Input: part model. Units: mm. Frame: model coordinates. Face numbers are marked on the shaded views. A direction names the side the tool comes from. Coordinates: 2 decimals unless noted, no trailing zeros. Write each loop counter-clockwise with the first axis right and the second up, starting at its lowest first coordinate (ties: lowest second). Pieces come first, ordered by that corner, then holes.
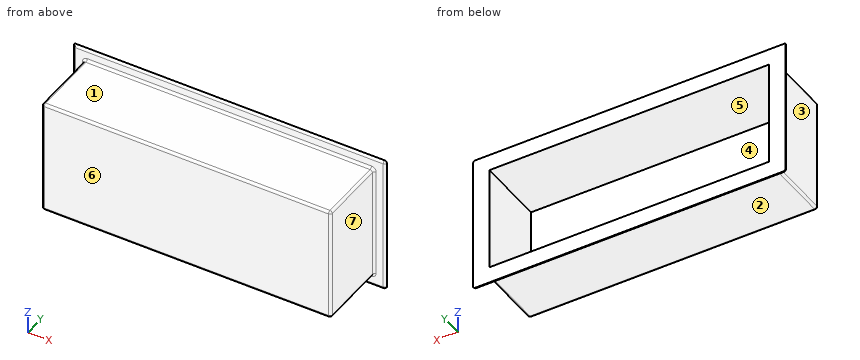
from build123d import *

# Parameters (mm, degrees)
F1_W        = 123
F1_H        = 49
F1_W_2      = 119
F1_H_2      = 45
F2_DEPTH    = 31
F1_H_3      = 5
F3_DEPTH    = 1
F4_DEPTH    = 31
F5_DEPTH    = 29
F6_F1_R     = 0.9999
F6_F2_R     = 1
F7_T1_DEPTH = 3.5
F7_T4_ANGLE = 90
F7_T6_ANGLE = 90
F7_T8_ANGLE = 90


# Not quite as in the source:
# - a fillet or chamfer that OpenCascade refuses, or shapes differently, is made with other operations: its cross-section is extruded or revolved along the edge and cut away or added
# - a fillet or chamfer is up to 0.001 mm smaller than in the source, because OpenCascade refuses the exact size


with BuildPart() as f2:
    # F1 (on offset) → F2 (new body)
    with BuildSketch(Plane.XZ.offset(15)):
        Rectangle(F1_W, F1_H)
        Rectangle(F1_W_2, F1_H_2, mode=Mode.SUBTRACT)
    extrude(amount=F2_DEPTH)

    # F1 (on offset) → F3 (join)
    with BuildSketch(Plane.XZ.offset(15)):
        with Locations((0, 27)):
            Rectangle(F1_W, F1_H_3)
        Polygon((-61.5, -29.5), (-61.5, -24.5), (-61.5, 24.5), (-61.5, 29.5), (-66.5, 29.5), (-66.5, -29.5), align=None)
        with Locations((0, -27)):
            Rectangle(F1_W, F1_H_3)
        Polygon((61.5, 24.5), (61.5, -24.5), (61.5, -29.5), (66.5, -29.5), (66.5, 29.5), (61.5, 29.5), align=None)
    extrude(amount=F3_DEPTH)

    # F1 (on offset) → F4 (join)
    with BuildSketch(Plane.XZ.offset(15)):
        Rectangle(F1_W_2, F1_H_2)
    extrude(amount=F4_DEPTH)

    # F1 (on offset) → F5 (cut)
    with BuildSketch(Plane.XZ.offset(15)):
        Rectangle(F1_W_2, F1_H_2)
    extrude(amount=F5_DEPTH, mode=Mode.SUBTRACT)

    # F6: fillet of radius 1 on 14 edges, made by hand

    # F6_f1 (radius 1 in the source; OpenCascade refuses exactly that, so slightly less here)
    f6_f1_edges = [f2.edges().sort_by_distance(p)[0] for p in [
        (61.5, -31, 24.5),
        (61.5, -31, -24.5),
        (61.5, -46, 0),
        (0, -46, -24.5),
        (0, -46, 24.5),
        (-61.5, -31, -24.5),
        (-61.5, -31, 24.5),
        (-61.5, -46, 0),
        (0, -16, -29.5),
        (-66.5, -16, 0),
        (0, -16, 29.5),
        (66.5, -16, 0),
    ]]
    fillet(f6_f1_edges, radius=F6_F1_R)

    # F6_f2
    f6_f2_edges = [f2.edges().sort_by_distance(p)[0] for p in [
        (61.5, -16, 0),
        (-61.5, -16, 0),
        (-61.2071360705, -16, -24.2071360705),
        (-61.2071360705, -16, 24.2071360705),
        (61.2071360705, -16, 24.2071360705),
        (61.2071360705, -16, -24.2071360705),
    ]]
    fillet(f6_f2_edges, radius=F6_F2_R)

    # F7: fillet of radius 1 on 7 edges, made by hand

    # F7_s2 → F7_t1 (cut)
    with BuildSketch(Plane.XZ.offset(12.5)):
        with BuildLine():
            ThreePointArc((-65.5, -29.5), (-66.2071067812, -29.2071067812), (-66.5, -28.5))
            Line((-66.5, -28.5), (-66.5, -29.5))
            Line((-66.5, -29.5), (-65.5, -29.5))
        make_face()
        with BuildLine():
            ThreePointArc((65.5, -29.5), (66.2071067812, -29.2071067812), (66.5, -28.5))
            Line((66.5, -28.5), (66.5, -29.5))
            Line((66.5, -29.5), (65.5, -29.5))
        make_face()
        with BuildLine():
            ThreePointArc((66.5, 28.5), (66.2071067812, 29.2071067812), (65.5, 29.5))
            Line((65.5, 29.5), (66.5, 29.5))
            Line((66.5, 29.5), (66.5, 28.5))
        make_face()
    extrude(amount=F7_T1_DEPTH, mode=Mode.SUBTRACT)

    # F7_s3 → F7_t4 (revolve, cut)
    with BuildSketch(Plane.XY.offset(-28.5)):
        with BuildLine():
            ThreePointArc((-65.5001, -16), (-66.2071360705, -15.7071360705), (-66.5, -15.0001))
            Line((-66.5, -15.0001), (-66.5, -16))
            Line((-66.5, -16), (-65.5001, -16))
        make_face()
    revolve(axis=Axis((-65.5, -16, -28.5), (0, -1, 0)), revolution_arc=F7_T4_ANGLE, mode=Mode.SUBTRACT)

    # F7_s5 → F7_t6 (revolve, cut)
    with BuildSketch(Plane.YZ.offset(65.5)):
        with BuildLine():
            ThreePointArc((-16, -28.5001), (-15.7071360705, -29.2071360705), (-15.0001, -29.5))
            Line((-15.0001, -29.5), (-16, -29.5))
            Line((-16, -29.5), (-16, -28.5001))
        make_face()
    revolve(axis=Axis((65.5, -16, -28.5), (0, -1, 0)), revolution_arc=F7_T6_ANGLE, mode=Mode.SUBTRACT)

    # F7_s7 → F7_t8 (revolve, cut)
    with BuildSketch(Plane.XY.offset(28.5)):
        with BuildLine():
            ThreePointArc((65.5001, -16), (66.2071360705, -15.7071360705), (66.5, -15.0001))
            Line((66.5, -15.0001), (66.5, -16))
            Line((66.5, -16), (65.5001, -16))
        make_face()
    revolve(axis=Axis((65.5, -16, 28.5), (0, -1, 0)), revolution_arc=F7_T8_ANGLE, mode=Mode.SUBTRACT)


solid = f2.part
Item 1: Pull-direction query (X, two-part tool) for the marked faces 5, 6 and 7; classes: released by +X, released by -X, zero draft, split by the parting line, or undercut.
Item 2: Section query A-A, the plane y = -26.5. Return loops of the section in (x, z).
Item 3: Material intervals for line 1 (X direction, y = -39, z = -5); line 2 (Z direction, x = 22, y = -31); line 3 (Y direction, x = 45, z = 1), sorted ascending.
Item 4: Pin query (flat end, axial travel): pin 1 Ø8.5 at (x, y) = (-0.5, -24.5) entering from +Z; pin 2 Ø4 at (x, z) = (44.5, -9) entering from +Y; pin 3 Ø3 at (y, z) = (-28, -23) entering from -X. Return the tip coordinate at first contact, or that it passes through.
Item 5: Access query for the marked faces 1, 2, 3 and 4. Directions: +Z, -Z, +X, -X, +Y, -Y. A direction counts if a zero-diameter tool reaches every point of the face in a straight line with its end or side. Return the directions, or none.
The answers:
1. face 5: undercut
1. face 6: zero draft
1. face 7: released by +X
2. outline: (-61.5, -23.5) arc R1 ccw to (-60.5, -24.5) - (60.5, -24.5) arc R1 ccw to (61.5, -23.5) - (61.5, 23.5) arc R1 ccw to (60.5, 24.5) - (-60.5, 24.5) arc R1 ccw to (-61.5, 23.5) - close; hole (-59.5, -22.5) - (59.5, -22.5) - (59.5, 22.5) - (-59.5, 22.5) - close
3. line 1: x = -61.5 to -59.5, 59.5 to 61.5
3. line 2: z = -24.5 to -22.5, 22.5 to 24.5
3. line 3: y = -46 to -44
4. pin 1: stops at z = 24.5
4. pin 2: stops at y = -44
4. pin 3: stops at x = -61.5
5. face 1: +Z, +X, -X, -Y
5. face 2: -Z, +X, -X, -Y
5. face 3: +Z, -Z, -X, -Y
5. face 4: +Y
